Read the model definition and answer for the solid it produces. Units are mm, in the model's axes. Face numbers are marked on the shaded views. Give positions to 0.01 mm unless a question says otherwise; leave off trailing zeros. Loops run counter-clockwise (first coordinate to the right, second up) from the corner with the lowest first, then second, coordinate; pieces in that order, holes last. Notation, with made-up numbers: (-18, -22) - (19, -22) arc R16 ccw to (19, -12) - close; hole circle Ø8 at (71, 83.25). An arc over 180 degrees is marked (long way). Write item = value, one per line. Start each with the question number.
from build123d import *

# Parameters (mm, degrees)
SKETCH1_W           = 25.4
SKETCH1_H           = 60.9287072
BOSS_EXTRUDE1_DEPTH = 1.5875


with BuildPart() as part:
    # Sketch1 → Boss-Extrude1 (new, symmetric)
    with BuildSketch(Plane.XY):
        Rectangle(SKETCH1_W, SKETCH1_H)
    extrude(amount=BOSS_EXTRUDE1_DEPTH, both=True)

    # Sketch3 → CSK for 1/4 Flat Head Machine Screw1 (revolve, cut)
    with BuildSketch(Plane(origin=(0, -17.7643536, 1.5875), x_dir=(0, -1, 0), z_dir=(1, 0, 0))):
        Polygon((0, 0), (0, 3.175), (3.3782, 3.175), (3.3782, 3.520932584), (6.4389, 0), align=None)
    revolve(axis=Axis((0, -17.7643536, 7.9375), (0, 0, -1)), mode=Mode.SUBTRACT)


solid = part.part
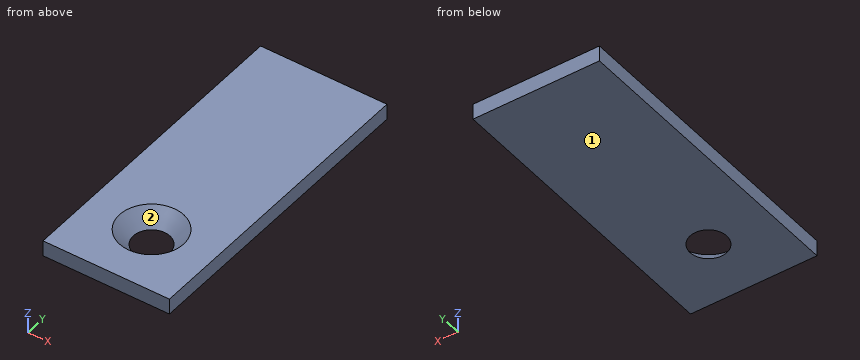
1. A cutting plane is placed at A-A on x = 0. Give the vertices of the cut face in (y, z).
2. A cutting plane is placed at B-B on z = -1.05. Give the vertices of the cut face in (x, y), and give its area (3 significant figures).
3. For a pull along Y with two mould halves and no side action, classify the marked faces 1 and 2 as released by +Y, released by -Y, zero draft, split by the parting line, or undercut.
4. Consider line 1 along Y through (x, z) = (3.25, 0.6); line 2 along X through (y, z) = (-21, -0.25); line 3 along Y through (x, z) = (1.25, 1.4). Determine where each line is inside the solid, lowest interval first. Write a range as [from, to].
Reply:
q1.outline = (-30.46, -1.59) - (-21.44, -1.59) - (-24.2, 1.59) - (-30.46, 1.59) - close; (-14.09, -1.59) - (30.46, -1.59) - (30.46, 1.59) - (-11.33, 1.59) - close
q2.outline = (-12.7, -30.46) - (12.7, -30.46) - (12.7, 30.46) - (-12.7, 30.46) - close; hole circle Ø8.29 at (0, -17.76)
q2.area = 1,490 mm^2
q3.face_1 = zero draft
q3.face_2 = undercut
q4.line_1 = [-30.46, -22.3], [-13.23, 30.46]
q4.line_2 = [-12.7, -3.6], [3.6, 12.7]
q4.line_3 = [-30.46, -23.91], [-11.61, 30.46]
